Source: CAD feature listing. Evaluate the final solid. Frame: model axes, mm. Round coordinates to 2 decimals unless told otherwise and drop trailing zeros. Write each loop counter-clockwise with the first axis right and the second up, starting at its lowest first coordinate (ties: lowest second). Pieces come first, ordered by that corner, then holes.
from build123d import *

# Parameters (mm, degrees)
F1_DEPTH = 72
F2_R     = 2


with BuildPart() as f1:
    # F0 (on Right) → F1 (new body)
    with BuildSketch(Plane.YZ):
        Polygon((20, 3.52654), (20, 0), (55, 0), (55, 9.697984), align=None)
    extrude(amount=F1_DEPTH)

    # F2
    f2_edges = [f1.edges().sort_by_distance(p)[0] for p in [
        (36, 55, 9.697984),
        (36, 20, 3.52654),
    ]]
    fillet(f2_edges, radius=F2_R)


solid = f1.part
1) Section query A-A on x = 18. Return the cut outline in (y, z), then the cut area to 3 significant figures.
Taken from the geometry:
outline: (20, 0) - (55, 0) - (55, 7.31) arc R2 ccw to (52.65, 9.28) - (21.65, 3.82) arc R2 ccw to (20, 1.85) - close
area: 230 mm2
2) Section query B-B on y = 26. Return the cut outline in (x, z), then the cut area to 3 significant figures.
Taken from the geometry:
outline: (0, 0) - (72, 0) - (72, 4.58) - (0, 4.58) - close
area: 330 mm2
3) Contact query for flat-ended pins moving along their axis: P1, Ø5, axis at x = 41.5, y = 40, coming from the -Z side; P2, Ø6, axis at x = 59.5, y = 42.5, coming from the +Z side. Output: stop coordinate, or through.
Taken from the geometry:
P1: stops at z = 0
P2: stops at z = 8.02
4) Material intervals for line 1 (Z direction, x = 12, y = 36); line 2 (Z direction, x = 53, y = 37); line 3 (Y direction, x = 56.5, z = 3.5), sorted ascending.
Taken from the geometry:
line 1: z = 0 to 6.35
line 2: z = 0 to 6.52
line 3: y = 20.87 to 55
5) Section query C-C on z = 6.25. Return the cut outline in (x, y).
Taken from the geometry:
outline: (0, 35.45) - (72, 35.45) - (72, 55) - (0, 55) - close
